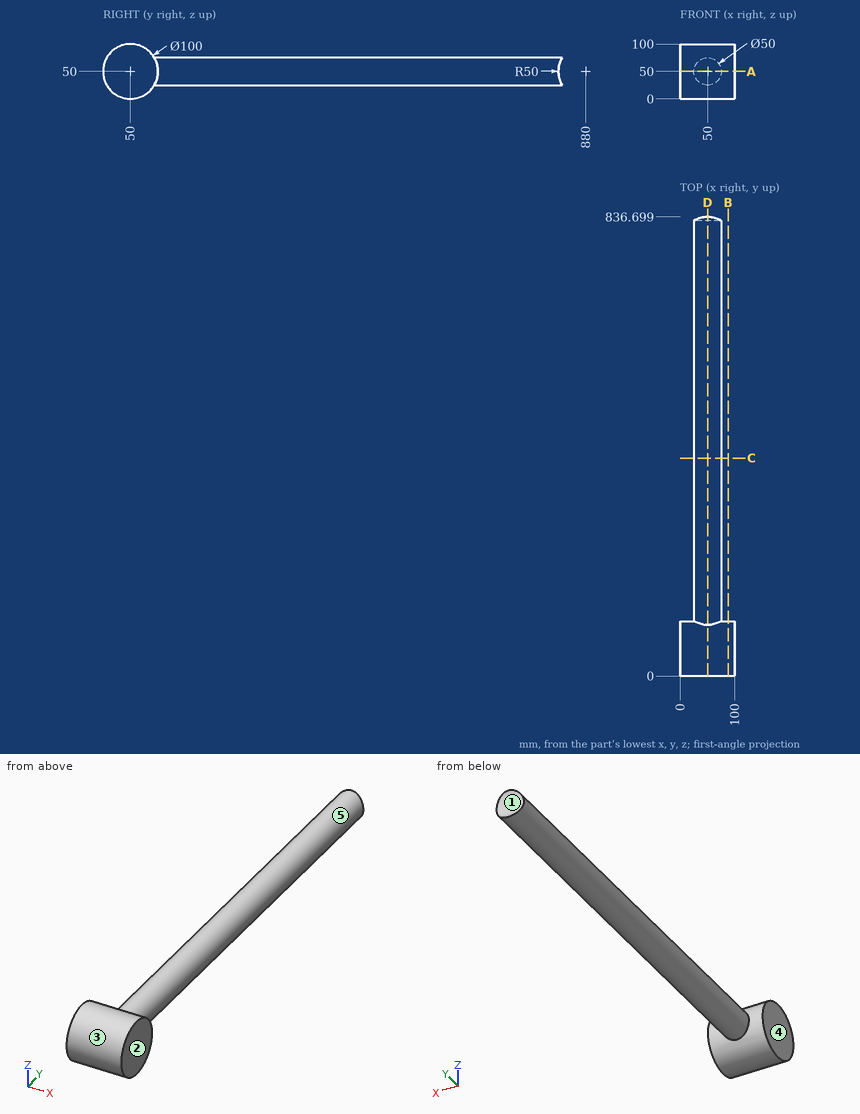
Geometry: see drawing. Coordinates: mm, zero at the bounding-box minimum. A direction names the side the tool comes from. Round coordinates to 2 decimals unless told otherwise and drop trailing zeros. Loops run counter-clockwise (first coordinate to the right, second up) from the corner with the lowest first, then second, coordinate; pieces in that order, holes last. Notation, with made-up numbers: M -20.75,-25.5 L 31.25,-25.5 A14 ccw 31.25,-21.5 Z; hole C -7,82 d4. An arc over 180 degrees is marked long. Use a Markdown table: item, result. Add a question column.
1. Reachability of the marked faces 4 and 5 from +Z, -Z, +X, -X, +Y, -Y: full face, straight path, thin tool, end or side. Return the list, or none.
2. Contact query for flat-ended pins moving along their axis: P1, Ø2, axis at y = 323.5, z = 59, coming from the +X side (1 decimal); P2, Ø2, axis at x = 76.5, y = 213.5, coming from the -Z side; P3, Ø12, axis at y = 588, z = 32.5, coming from the -X side; P4, Ø1, axis at x = 43, z = 11.5, coming from the +Y side (1 decimal). Output: stop coordinate, or through.
3. Section query B-B on x = 87.5. Return the cut outline in (y, z).
4. Mould query, pull axis Z, two halves, no side actions, for the marked faces 1, 2 and 3. Classes: pulls with the +Z half, pulls with the -Z half, needs draft (parallel to the pull), parting line crosses it, or undercut.
5. Line query: line 1 (Y direction, x = 93.5, z = 46); line 2 (Y direction, x = 68.5, z = 69); line 3 (Z direction, x = 36.5, y = 613). Output: solid intervals per line, ascending.
6. Section query C-C on y = 397. Return the cut outline in (x, z), then the cut area to 3 significant figures.
7. Section query D-D on x = 50. Return the cut outline in (y, z), then the cut area to 3 significant figures.
8. Section query A-A on z = 50. Return the cut outline in (x, y), then the cut area to 3 significant figures.
Reported:
| question | item | result |
|---|---|---|
| 1 | face 4 | +Z, -Z, -X, +Y, -Y |
| 1 | face 5 | +Y |
| 2 | P1 | stops at x = 73.7 |
| 2 | P2 | passes through |
| 2 | P3 | stops at x = 27.8 |
| 2 | P4 | stops at y = 82.5 |
| 3 | outline | C 50,50 d100 |
| 4 | face 1 | undercut |
| 4 | face 2 | needs draft |
| 4 | face 3 | parting line crosses it |
| 5 | line 1 | y = 0.16 to 99.84 |
| 5 | line 2 | y = 3.75 to 96.25 |
| 5 | line 3 | z = 28.96 to 71.04 |
| 6 | outline | C 50,50 d50 |
| 6 | area | 1,960 mm² |
| 7 | outline | M 93.3,25 L 836.7,25 A50 cw 836.7,75 L 93.3,75 A50 ccw long Z |
| 7 | area | 44,600 mm² |
| 8 | outline | M 0,0 L 100,0 L 100,100 L 75,100 L 75,830 L 25,830 L 25,100 L 0,100 Z |
| 8 | area | 46,500 mm² |
